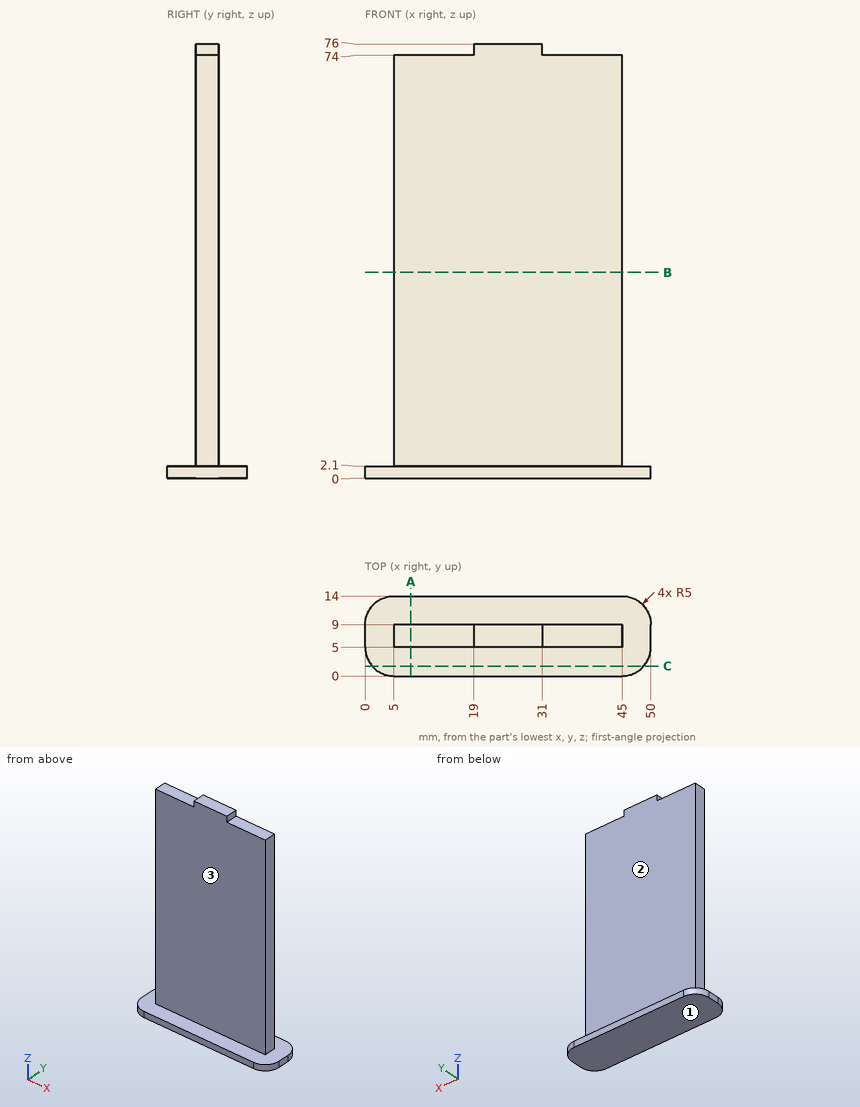
Geometry check sheet. Reference: drawing and pictorial views, mm from the part's lowest x, y, z. A direction names the side the tool comes from. Round coordinates to 2 decimals unless told otherwise and drop trailing zeros. Order: outer loops, then holes, each group sorted by start corner. A loop starts at its lowest first (then second) coordinate and runs counter-clockwise, first axis right, second up.
Q1. Set-up check for the marked faces 1, 2 and 3: record each of +Z, -Z, +X, -X, +Y, -Y from which the full face is reachable in a straight line by a thin tool's end or side.
Filled sheet:
face 1: -Z, +X, -X, +Y, -Y
face 2: +Z, +X, -X, +Y
face 3: +Z, +X, -X, -Y
Q2. Cross-section at A-A, the plane x = 8. Enter the section's corners in (y, z), plus the area to 3 significant figures.
Filled sheet:
outline: (0, 0) - (14, 0) - (14, 2.1) - (9, 2.1) - (9, 74) - (5, 74) - (5, 2.1) - (0, 2.1) - close
area: 317 mm2
Q3. Depth check by flat-ended pin: P1, Ø3, axis at x = 10.5, y = 7, coming from the +Z side; P2, Ø6, axis at x = 40, z = 47, coming from the -Y side; P3, Ø3, axis at y = 7.5, z = 39, coming from the +X side; P4, Ø8, axis at x = 20, y = 12, coming from the +Z side. Enter the tip coordinate at first touch or a pass-through.
Filled sheet:
P1: stops at z = 74
P2: stops at y = 5
P3: stops at x = 45
P4: stops at z = 76
Q4. Cross-section at B-B, the plane z = 36. Enter the section's corners in (x, y), plus the area to 3 significant figures.
Filled sheet:
outline: (5, 5) - (45, 5) - (45, 9) - (5, 9) - close
area: 160 mm2
Q5. Scan lines: L1, parallel to X at y = 6, z = 4.5; L2, parallel to Y at x = 13, z = 53; L3, parallel to Z at x = 35.5, y = 8. Record each from-to range of solid material in increasing order.
Filled sheet:
L1: x = 5 to 45
L2: y = 5 to 9
L3: z = 0 to 74
Q6. Cross-section at C-C, the plane y = 1.75. Enter the section's corners in (x, z), plus the area to 4 significant figures.
Filled sheet:
outline: (1.2, 0) - (48.8, 0) - (48.8, 2.1) - (1.2, 2.1) - close
area: 100.0 mm2
